Could you check a few things on this model? Use its own coordinates, in mm. A direction names the side the tool comes from. Give positions to 0.01 mm unless a question says otherwise; leave off trailing zeros. Order: outer loops, then holes, each group sorted by start corner. A loop starts at its lowest first (then second) coordinate and runs counter-clockwise, first axis right, second up. Notation, with made-up numbers: M 84.5,63.5 L 111.5,63.5 A11 cw 111.5,72.5 Z; hole C 29,7.25 d8. An arc over 180 degrees is marked long. Answer in a Markdown table with one row per item. Add a question column.
```python
from build123d import *

# Parameters (mm, degrees)
SKETCH1_W                     = 41.91
SKETCH1_H                     = 32.385
BOSS_EXTRUDE1_DEPTH           = 1.651
SKETCH2_R                     = 1.524
CUT_EXTRUDE1_DEPTH            = 27.533655652
SKETCH3_W                     = 5.08
SKETCH3_H                     = 0.889
BOSS_EXTRUDE2_DEPTH           = 1.905
BOSS_EXTRUDE3_DEPTH           = 1.905
BOSS_EXTRUDE3_DEPTH_BACK      = 6.35
SKETCH4_W                     = 2.286
SKETCH4_H                     = 9.017
SKETCH5_R                     = 2.54
BOSS_EXTRUDE4_DEPTH           = 7.62
SKETCH6_W                     = 2.54
SKETCH6_H                     = 7.9375
BOSS_EXTRUDE5_DEPTH           = 2.54
SKETCH7_W                     = 0.635
SKETCH7_H                     = 0.635
BOSS_EXTRUDE6_DEPTH           = 7.62
SKETCH8_W                     = 0.635
SKETCH8_H                     = 0.635
BOSS_EXTRUDE7_DEPTH           = 0.635
BOSS_EXTRUDE7_DRAFT           = 20
BOSS_EXTRUDE7_PROFILE_2_DEPTH = 0.635
BOSS_EXTRUDE7_PROFILE_2_DRAFT = 20
BOSS_EXTRUDE7_PROFILE_3_DEPTH = 0.635
BOSS_EXTRUDE7_PROFILE_3_DRAFT = 20


with BuildPart() as part:
    # Sketch1 → Boss-Extrude1 (new body)
    with BuildSketch(Plane(origin=(0, 0, 0), x_dir=(1, 0, 0), z_dir=(0, 1, 0))):
        Rectangle(SKETCH1_W, SKETCH1_H)
    extrude(amount=BOSS_EXTRUDE1_DEPTH)

    # Sketch2 → Cut-Extrude1 (cut, through all)
    with BuildSketch(Plane(origin=(0, 1.651, 0), x_dir=(1, 0, 0), z_dir=(0, 1, 0))):
        with Locations(Location((-16.891, 12.1285, 0), (0, 0, 270))):
            Circle(SKETCH2_R)
        with Locations(Location((16.891, 12.1285, 0), (0, 0, 270))):
            Circle(SKETCH2_R)
        with Locations(Location((-16.891, -12.1285, 0), (0, 0, 270))):
            Circle(SKETCH2_R)
        with Locations(Location((16.891, -12.1285, 0), (0, 0, 270))):
            Circle(SKETCH2_R)
    extrude(amount=-CUT_EXTRUDE1_DEPTH, mode=Mode.SUBTRACT)

    # Sketch3 → Boss-Extrude2 (add)
    with BuildSketch(Plane(origin=(0, 1.651, 0), x_dir=(1, 0, 0), z_dir=(0, 1, 0))):
        with Locations((18.415, 4.064)):
            Rectangle(SKETCH3_W, SKETCH3_H)
        with Locations((18.415, -4.064)):
            Rectangle(SKETCH3_W, SKETCH3_H)
    extrude(amount=BOSS_EXTRUDE2_DEPTH)

    # Sketch4 → Boss-Extrude3 (add, two sides: drawn at the far end of the back side and taken through both)
    with BuildSketch(Plane(origin=(0, 1.651, 0), x_dir=(1, 0, 0), z_dir=(0, 1, 0)).offset(-BOSS_EXTRUDE3_DEPTH_BACK)):
        with Locations((22.098, 0)):
            Rectangle(SKETCH4_W, SKETCH4_H)
    extrude(amount=BOSS_EXTRUDE3_DEPTH + BOSS_EXTRUDE3_DEPTH_BACK)

    # Sketch5 → Boss-Extrude4 (add)
    with BuildSketch(Plane(origin=(23.241, 0, 0), x_dir=(0, 0, -1), z_dir=(1, 0, 0))):
        with Locations(Location((0, -0.5715, 0), (0, 0, 180))):
            Circle(SKETCH5_R)
    extrude(amount=BOSS_EXTRUDE4_DEPTH)

    # Sketch6 → Boss-Extrude5 (add)
    with BuildSketch(Plane.XZ):
        with Locations((-17.145, 0)):
            Rectangle(SKETCH6_W, SKETCH6_H)
    extrude(amount=BOSS_EXTRUDE5_DEPTH)

    # Sketch7 → Boss-Extrude6 (add)
    with BuildSketch(Plane.ZY.offset(18.415)):
        with Locations((1.984375, -1.27)):
            Rectangle(SKETCH7_W, SKETCH7_H)
        with Locations((0, -1.27)):
            Rectangle(SKETCH7_W, SKETCH7_H)
        with Locations((-1.984375, -1.27)):
            Rectangle(SKETCH7_W, SKETCH7_H)
    extrude(amount=BOSS_EXTRUDE6_DEPTH)


with BuildPart() as boss_extrude7_tool:
    # Sketch8 → Boss-Extrude7 (with draft: the straight prism first)
    with BuildSketch(Plane.ZY.offset(26.035)):
        with Locations((-1.984375, -1.27)):
            Rectangle(SKETCH8_W, SKETCH8_H)
    extrude(amount=BOSS_EXTRUDE7_DEPTH)
    # Boss-Extrude7: the draft: its side faces are tilted about the plane it starts from
    boss_extrude7_sides = [boss_extrude7_tool.faces().sort_by_distance(p)[0] for p in [
        (-26.3525, -1.27, -2.301875),
        (-26.3525, -1.5875, -1.984375),
        (-26.3525, -1.27, -1.666875),
        (-26.3525, -0.9525, -1.984375),
    ]]
    draft(boss_extrude7_sides, Plane.ZY.offset(26.035), BOSS_EXTRUDE7_DRAFT)


with BuildPart() as part_1:
    add(part.part)

    # Boss-Extrude7: add boss_extrude7_tool
    add(boss_extrude7_tool.part)


with BuildPart() as boss_extrude7_profile_2_tool:
    # Sketch8 → Boss-Extrude7 profile 2 (with draft: the straight prism first)
    with BuildSketch(Plane.ZY.offset(26.035)):
        with Locations((0, -1.27)):
            Rectangle(SKETCH8_W, SKETCH8_H)
    extrude(amount=BOSS_EXTRUDE7_PROFILE_2_DEPTH)
    # Boss-Extrude7 profile 2: the draft: its side faces are tilted about the plane it starts from
    boss_extrude7_profile_2_sides = [boss_extrude7_profile_2_tool.faces().sort_by_distance(p)[0] for p in [
        (-26.3525, -1.27, -0.3175),
        (-26.3525, -1.5875, 0),
        (-26.3525, -1.27, 0.3175),
        (-26.3525, -0.9525, 0),
    ]]
    draft(boss_extrude7_profile_2_sides, Plane.ZY.offset(26.035), BOSS_EXTRUDE7_PROFILE_2_DRAFT)


with BuildPart() as part_2:
    add(part_1.part)

    # Boss-Extrude7 profile 2: add boss_extrude7_profile_2_tool
    add(boss_extrude7_profile_2_tool.part)


with BuildPart() as boss_extrude7_profile_3_tool:
    # Sketch8 → Boss-Extrude7 profile 3 (with draft: the straight prism first)
    with BuildSketch(Plane.ZY.offset(26.035)):
        with Locations((1.984375, -1.27)):
            Rectangle(SKETCH8_W, SKETCH8_H)
    extrude(amount=BOSS_EXTRUDE7_PROFILE_3_DEPTH)
    # Boss-Extrude7 profile 3: the draft: its side faces are tilted about the plane it starts from
    boss_extrude7_profile_3_sides = [boss_extrude7_profile_3_tool.faces().sort_by_distance(p)[0] for p in [
        (-26.3525, -1.27, 1.666875),
        (-26.3525, -1.5875, 1.984375),
        (-26.3525, -1.27, 2.301875),
        (-26.3525, -0.9525, 1.984375),
    ]]
    draft(boss_extrude7_profile_3_sides, Plane.ZY.offset(26.035), BOSS_EXTRUDE7_PROFILE_3_DRAFT)


with BuildPart() as part_3:
    add(part_2.part)

    # Boss-Extrude7 profile 3: add boss_extrude7_profile_3_tool
    add(boss_extrude7_profile_3_tool.part)


solid = part_3.part
```
1. Will these pins go through, and if not, where does the flat tip stop? P1, Ø1.5, axis at y = 2.5, z = -1, coming from the -X side (3 decimals); P2, Ø12, axis at x = -20, z = 5, coming from the +Y side; P3, Ø5, axis at x = 4.5, z = 12.5, coming from the -Y side; P4, Ø1.5, axis at x = 1.5, y = 2, coming from the -Z side.
2. If I drill on line 1 along X through (y, z) = (0.5, -11) (3 decimals); line 2 along Y through (x, z) = (-18.5, 0); line 3 along Y through (x, z) = (20.5, 1), over which ranges is the centre line in solid material (lowest first)? Write a range as [from, to].
3. Suppose I cut it at D-D on x = -1. List the corners of the cut face in (y, z) for me.
4. For faces 1 (the flat face through (18, 3, -3.62)), 2 (the cylindrical face through (-18.38, 0.84, 11.8)), 3 (the flat face through (-17, -2.54, 0)), 4 (the flat face through (20.955, -2, 0)), which set-ups out of +Z, -Z, +X, -X, +Y, -Y let a thin tool reach every point of the face, with its end or its side?
5. Suppose I cut it at A-A on x = -23. List the corners of the cut face in (y, z) for me, plus the area to 3 significant figures.
6. Suppose I cut it at C-C on y = 0.75. List the corners of the cut face in (x, z) for me (1 decimal).
7. Thinking about a two-plate mould opening in Z: for faces 5 (the cylindrical face through (16.958, 0.837, 10.606)), 6 (the flat face through (-17, -1, 3.969)), 7 (the flat face through (21.14, 3.556, -0.06)), which applies, pulls with the +Z half, pulls with the -Z half, needs draft (parallel to the pull), parting line crosses it, or undercut?
8. Suppose I cut it at B-B on z = 11.5. List the corners of the cut face in (x, y) for me (3 decimals).
Findings below:
| question | item | result |
|---|---|---|
| 1 | P1 | x = 20.955 |
| 1 | P2 | y = 1.65 |
| 1 | P3 | y = 0 |
| 1 | P4 | z = -16.19 |
| 2 | line 1 | [-20.955, -17.915], [-15.867, 15.867], [17.915, 20.955] |
| 2 | line 2 | [-1.59, -0.95], [0, 1.65] |
| 2 | line 3 | [0, 1.65] |
| 3 | outline | M 0,-16.19 L 1.65,-16.19 L 1.65,16.19 L 0,16.19 Z |
| 4 | face 1 | -X, +Y |
| 4 | face 2 | +Y, -Y |
| 4 | face 3 | +Z, -Z, -X, -Y |
| 4 | face 4 | +Z, -Z, -Y |
| 5 | outline | M -1.59,-2.3 L -0.95,-2.3 L -0.95,-1.67 L -1.59,-1.67 Z; M -1.59,-0.32 L -0.95,-0.32 L -0.95,0.32 L -1.59,0.32 Z; M -1.59,1.67 L -0.95,1.67 L -0.95,2.3 L -1.59,2.3 Z |
| 5 | area | 1.21 mm2 |
| 6 | outline | M -21,-16.2 L 21,-16.2 L 21,-4.5 L 23.2,-4.5 L 23.2,-2.2 L 30.9,-2.2 L 30.9,2.2 L 23.2,2.2 L 23.2,4.5 L 21,4.5 L 21,16.2 L -21,16.2 Z; hole C -16.9,-12.1 d3; hole C -16.9,12.1 d3; hole C 16.9,-12.1 d3; hole C 16.9,12.1 d3 |
| 7 | face 5 | undercut |
| 7 | face 6 | pulls with the +Z half |
| 7 | face 7 | needs draft |
| 8 | outline | M -20.955,0 L -18.279,0 L -18.279,1.651 L -20.955,1.651 Z; M -15.503,0 L 15.503,0 L 15.503,1.651 L -15.503,1.651 Z; M 18.279,0 L 20.955,0 L 20.955,1.651 L 18.279,1.651 Z |
